Source: CAD feature listing. Evaluate the final solid. Frame: model axes, mm. A direction names the side the tool comes from. Give positions to 0.01 mm unless a question says otherwise; leave off trailing zeros. Order: outer loops, then holes, each group sorted by start corner. A loop starts at its lowest first (then second) coordinate and runs counter-clockwise, first axis right, second up.
```python
from build123d import *

# Parameters (mm, degrees)
SKETCH1_R           = 13
BOSS_EXTRUDE1_DEPTH = 2.3
SKETCH2_R           = 0.5
BOSS_EXTRUDE2_DEPTH = 15


with BuildPart() as part:
    # Sketch1 → Boss-Extrude1 (new, symmetric)
    with BuildSketch(Plane.XY):
        Circle(SKETCH1_R)
    extrude(amount=BOSS_EXTRUDE1_DEPTH, both=True)

    # Sketch2 → Boss-Extrude2 (add)
    with BuildSketch(Plane(origin=(0, 0, 0), x_dir=(1, 0, 0), z_dir=(0, 1, 0))):
        with Locations(Location((-5, 0, 0), (0, 0, 270))):
            Circle(SKETCH2_R)
        with Locations(Location((5, 0, 0), (0, 0, 270))):
            Circle(SKETCH2_R)
    extrude(amount=-BOSS_EXTRUDE2_DEPTH)


solid = part.part
```
1) Section query D-D, the plane z = -1.35. Return the cut outline in (x, y).
Report:
outline: circle Ø26 at (0, 0)
2) Material intervals for L1, parallel to Y at x = 0, z = -1.2; L2, parallel to Y at x = 2, z = -1.25; L3, parallel to X at y = 8.75, z = 1.3, sorted ascending.
Report:
L1: y = -13 to 13
L2: y = -12.85 to 12.85
L3: x = -9.61 to 9.61
3) Pin query (flat end, axial travel): pin 1 (2 mm diameter, centred on x = -6.5, z = -1.5, fed in from -Y). Return the tip coordinate at first contact, or that it passes through.
Report:
pin 1: stops at y = -11.78
4) Reachability of faces 3 (the cylindrical face through (5.496, -13.367, -0.065)), 4 (the flat face through (5, -15, 0)) from +Z, -Z, +X, -X, +Y, -Y: full face, straight path, thin tool, end or side. Return the list, or none.
Report:
face 3: -Y
face 4: +Z, -Z, +X, -X, -Y
5) Section query A-A, the plane x = 5. Return the cut outline in (y, z), and give its area (3 significant figures).
Report:
outline: (-15, -0.5) - (-12, -0.5) - (-12, -2.3) - (12, -2.3) - (12, 2.3) - (-12, 2.3) - (-12, 0.5) - (-15, 0.5) - close
area: 113 mm2
6) Section query B-B, the plane z = 0. Return the cut outline in (x, y).
Report:
outline: (-5.5, -15) - (-4.5, -15) - (-4.5, -12.2) arc R13 ccw to (4.5, -12.2) - (4.5, -15) - (5.5, -15) - (5.5, -11.78) arc R13 ccw (long way) to (-5.5, -11.78) - close
7) Draft query along X for faces 1 (the cylindrical face through (-5.444, -13.367, 0.231)), 2 (the flat face through (0, 0, -2.3)). Return one class per face: +X half, -X half, draft (parallel to the pull), parting line (faces both ways), or undercut.
Report:
face 1: undercut
face 2: draft
8) Section query C-C, the plane y = -4.75. Return the cut outline in (x, z), and give its area (3 significant figures).
Report:
outline: (-12.1, -2.3) - (12.1, -2.3) - (12.1, 2.3) - (-12.1, 2.3) - close
area: 111 mm2
